Could you check a few things on this model? Use its own coordinates, in mm. A direction names the side the tool comes from. Give positions to 0.01 mm unless a question says otherwise; leave off trailing zeros. Order: outer loops, then holes, each group sorted by start corner. A loop starts at its lowest first (then second) coordinate and runs counter-clockwise, first axis right, second up. Notation, with made-up numbers: (-26.75, 73.25) -> (20.25, 73.25) arc R18 ccw to (20.25, 91.25) -> close; hole circle Ø3 at (2, 4.5). An arc over 180 degrees is marked (long way). Answer as CSV lines item,"result". Start each with the question number.
(1) I want a section at A-A (x = 32). Give the number of separate pieces and of enclosed holes in the cut face, plus the area to 3 significant figures.
(2) On a 3-axis mill with a long thin cutter (end or side, diameter ignored), from which of +Z, -Z, +X, -X, +Y, -Y can I reach the whole of each face in a straight line? I mean faces 1 (the face through (63, 7, 0)), 2 (the face through (2.6, 7, -2)), 3 (the face through (32, 11, 41)), 4 (the face through (45.997, 8.731, 41.789)), 5 (the face through (61.4, 7, 42)). Say none if no direction works.
(3) Will these pins go through, and if not, where does the flat tip stop? pin 1 Ø5 at (x, z) = (38, 33) entering from +Y; pin 2 Ø1.3 at (y, z) = (5, -1) entering from +X; pin 3 Ø5 at (y, z) = (1.5, 18.5) entering from +X; pin 4 Ø1.5 at (y, z) = (1.5, 11) entering from -X.
(4) I want a section at D-D (x = 40). Please give me the cut outline in (y, z), plus the area to 3 significant figures.
(5) I need wall thicknesses on L1, parallel to Z at x = 63, y = 8.1; L2, parallel to Z at x = 44, y = 11.5; L3, parallel to X at y = 12, z = 23.5. Which ranges of each line are inside material? Lowest first, please.
(6) I want a section at B-B (z = 33). Please give me the cut outline in (x, y), plus the area to 3 significant figures.
(7) We'd pull the mould along Z, two halves only. Please class faces 6 (the face through (18.1, 8.19, 41.79)), 7 (the face through (32, 11, -2.6)), 8 (the face through (31.6, 1.6, 10.8)): released by +Z, released by -Z, zero draft, split by the parting line, or undercut.
(8) I want a section at C-C (y = 4.5). Please give me the cut outline in (x, z), plus the area to 3 significant figures.
```python
from build123d import *

# Parameters (mm, degrees)
SKETCH1_W                      = 64
SKETCH1_H                      = 40
BOSS_EXTRUDE1_DEPTH            = 1.6
SKETCH2_R                      = 2.1
CUT_EXTRUDE1_DEPTH             = 76.488807117
LPATTERN1_COUNT                = 2
LPATTERN1_PITCH                = 48
LPATTERN1_COUNT_DIR2           = 5
LPATTERN1_PITCH_DIR2           = 8
EDGE_FLANGE1_STRIP_W           = 8.4
EDGE_FLANGE1_STRIP_H           = 1.6
EDGE_FLANGE1_STRIP_CUT_DEPTH   = 40
EDGE_FLANGE1_STRIP_2_W         = 8.4
EDGE_FLANGE1_STRIP_2_H         = 1.6
EDGE_FLANGE1_STRIP_CUT_2_DEPTH = 40
EDGE_FLANGE1_DEPTH             = 40
EDGE_FLANGE1_BEND_DEPTH        = 40
SKETCH14_R                     = 2.1
CUT_EXTRUDE2_DEPTH             = 77.852130745
LPATTERN2_COUNT                = 5
LPATTERN2_PITCH                = 8
EDGE_FLANGE2_DEPTH             = 58.8
EDGE_FLANGE2_BEND_DEPTH        = 58.8
SKETCH25_R                     = 2.1
CUT_EXTRUDE3_DEPTH             = 80.700690085
LPATTERN3_COUNT                = 7
LPATTERN3_PITCH                = 8
SKETCH26_R                     = 9
SKETCH26_R_2                   = 2
CUT_EXTRUDE4_DEPTH             = 79.255479041


# Sheet-metal steps are written as plain solids
with BuildPart() as part:
    # Sketch1 → Boss-Extrude1 (new body)
    with BuildSketch(Plane(origin=(0, 0, 0), x_dir=(1, 0, 0), z_dir=(0, 1, 0))):
        with Locations((32, -20)):
            Rectangle(SKETCH1_W, SKETCH1_H)
    extrude(amount=BOSS_EXTRUDE1_DEPTH)

    # Sketch2 → Cut-Extrude1 (cut, through all)
    with BuildSketch(Plane(origin=(0, 1.6, 0), x_dir=(1, 0, 0), z_dir=(0, 1, 0))):
        with Locations(Location((8, -4, 0), (0, 0, 270))):
            Circle(SKETCH2_R)
    cut_extrude1 = extrude(amount=-CUT_EXTRUDE1_DEPTH, mode=Mode.SUBTRACT)

    # LPattern1: Cut-Extrude1 2 × 5
    with Locations(*[(i * LPATTERN1_PITCH, 0, j * LPATTERN1_PITCH_DIR2) for i in range(LPATTERN1_COUNT) for j in range(LPATTERN1_COUNT_DIR2) if (i, j) != (0, 0)]):
        add(cut_extrude1, mode=Mode.SUBTRACT)

    # Edge-Flange1 strip (across the edge) → Edge-Flange1 strip cut (cut)
    with BuildSketch(Plane(origin=(64, 1.6, 40), x_dir=(-1, 0, 0), z_dir=(0, 0, -1))):
        with Locations((-1.6, -0.8)):
            Rectangle(EDGE_FLANGE1_STRIP_W, EDGE_FLANGE1_STRIP_H)
    extrude(amount=EDGE_FLANGE1_STRIP_CUT_DEPTH, mode=Mode.SUBTRACT)

    # Edge-Flange1 strip 2 (across the edge) → Edge-Flange1 strip cut 2 (cut)
    with BuildSketch(Plane(origin=(0, 1.6, 0), x_dir=(1, 0, 0), z_dir=(0, 0, 1))):
        with Locations((-1.6, -0.8)):
            Rectangle(EDGE_FLANGE1_STRIP_2_W, EDGE_FLANGE1_STRIP_2_H)
    extrude(amount=EDGE_FLANGE1_STRIP_CUT_2_DEPTH, mode=Mode.SUBTRACT)

    # Edge-Flange1 section (across the edge) → Edge-Flange1 (add)
    with BuildSketch(Plane(origin=(64, 1.6, 40), x_dir=(-1, 0, 0), z_dir=(0, 0, -1))):
        with BuildLine():
            Line((0, 1), (0, 12.9))
            Line((0, 12.9), (1.6, 12.9))
            Line((1.6, 12.9), (1.6, 1))
            ThreePointArc((1.6, 1), (1.892893219, 0.292893219), (2.6, 0))
            Line((2.6, 0), (2.6, -1.6))
            ThreePointArc((2.6, -1.6), (0.761522369, -0.838477631), (0, 1))
        make_face()
    extrude(amount=EDGE_FLANGE1_DEPTH)

    # Edge-Flange1 section 2 (across the edge) → Edge-Flange1 bend (add)
    with BuildSketch(Plane(origin=(0, 1.6, 0), x_dir=(1, 0, 0), z_dir=(0, 0, 1))):
        with BuildLine():
            Line((0, 1), (0, 12.9))
            Line((0, 12.9), (1.6, 12.9))
            Line((1.6, 12.9), (1.6, 1))
            ThreePointArc((1.6, 1), (1.892893219, 0.292893219), (2.6, 0))
            Line((2.6, 0), (2.6, -1.6))
            ThreePointArc((2.6, -1.6), (0.761522369, -0.838477631), (0, 1))
        make_face()
    extrude(amount=EDGE_FLANGE1_BEND_DEPTH)

    # Sketch14 → Cut-Extrude2 (cut, through all)
    with BuildSketch(Plane.ZY):
        with Locations(Location((4, 8.1, 0), (0, 0, 270))):
            Circle(SKETCH14_R)
    cut_extrude2 = extrude(amount=-CUT_EXTRUDE2_DEPTH, mode=Mode.SUBTRACT)

    # LPattern2: Cut-Extrude2 ×5
    with Locations(*[(0, 0, i * LPATTERN2_PITCH) for i in range(1, LPATTERN2_COUNT)]):
        add(cut_extrude2, mode=Mode.SUBTRACT)

    # Edge-Flange2 section (across the edge) → Edge-Flange2 (add)
    with BuildSketch(Plane(origin=(2.6, 1.6, 41), x_dir=(0, 0, -1), z_dir=(1, 0, 0))):
        with BuildLine():
            Line((-1.6, 1), (-1.6, 13))
            Line((-1.6, 13), (0, 13))
            Line((0, 13), (0, 1))
            ThreePointArc((0, 1), (0.292893219, 0.292893219), (1, 0))
            Line((1, 0), (1, -1.6))
            ThreePointArc((1, -1.6), (-0.838477631, -0.838477631), (-1.6, 1))
        make_face()
    extrude(amount=EDGE_FLANGE2_DEPTH)

    # Edge-Flange2 section 2 (across the edge) → Edge-Flange2 bend (add)
    with BuildSketch(Plane(origin=(61.4, 1.6, -1), x_dir=(0, 0, 1), z_dir=(-1, 0, 0))):
        with BuildLine():
            Line((-1.6, 1), (-1.6, 13))
            Line((-1.6, 13), (0, 13))
            Line((0, 13), (0, 1))
            ThreePointArc((0, 1), (0.292893219, 0.292893219), (1, 0))
            Line((1, 0), (1, -1.6))
            ThreePointArc((1, -1.6), (-0.838477631, -0.838477631), (-1.6, 1))
        make_face()
    extrude(amount=EDGE_FLANGE2_BEND_DEPTH)

    # Sketch25 → Cut-Extrude3 (cut, through all)
    with BuildSketch(Plane(origin=(0, 0, -2.6), x_dir=(-1, 0, 0), z_dir=(0, 0, -1))):
        with Locations((-8, 8.1)):
            Circle(SKETCH25_R)
    cut_extrude3 = extrude(amount=-CUT_EXTRUDE3_DEPTH, mode=Mode.SUBTRACT)

    # LPattern3: Cut-Extrude3 ×7
    with Locations(*[(i * LPATTERN3_PITCH, 0, 0) for i in range(1, LPATTERN3_COUNT)]):
        add(cut_extrude3, mode=Mode.SUBTRACT)

    # Sketch26 → Cut-Extrude4 (cut, through all)
    with BuildSketch(Plane.XZ):
        with Locations(Location((32, 20, 0), (0, 0, 270))):
            Circle(SKETCH26_R)
        with Locations(Location((45, 20, 0), (0, 0, 270))):
            Circle(SKETCH26_R_2)
        with Locations(Location((32, 7, 0), (0, 0, 270))):
            Circle(SKETCH26_R_2)
        with Locations(Location((19, 20, 0), (0, 0, 270))):
            Circle(SKETCH26_R_2)
        with Locations(Location((32, 33, 0), (0, 0, 270))):
            Circle(SKETCH26_R_2)
    extrude(amount=-CUT_EXTRUDE4_DEPTH, mode=Mode.SUBTRACT)


solid = part.part
```
Final values:
1,separate pieces,"6"
1,enclosed holes,"0"
1,area,"56.4 mm²"
2,face 1,"-Z, +X, +Y, -Y"
2,face 2,"-Z, -X, +Y, -Y"
2,face 3,"+X, -X, +Y"
2,face 4,"+Z, -Z"
2,face 5,"+Z, +X, +Y, -Y"
3,pin 1,"y = 1.6"
3,pin 2,"x = 61.4"
3,pin 3,"x = 64"
3,pin 4,"x = 0.02"
4,outline,"(0, 0) arc R2.6 ccw to (2.6, -2.6) -> (6, -2.6) -> (6, -1) -> (2.6, -1) arc R1 cw to (1.6, 0) -> (1.6, 15.88) -> (0, 15.88) -> close; (0, 24.12) -> (1.6, 24.12) -> (1.6, 40) arc R1 cw to (2.6, 41) -> (6, 41) -> (6, 42.6) -> (2.6, 42.6) arc R2.6 ccw to (0, 40) -> close; (10.2, -2.6) -> (14.6, -2.6) -> (14.6, -1) -> (10.2, -1) -> close; (10.2, 41) -> (14.6, 41) -> (14.6, 42.6) -> (10.2, 42.6) -> close"
4,area,"84.8 mm²"
5,L1,"0 to 1.9, 6.1 to 9.9, 14.1 to 17.9, 22.1 to 25.9, 30.1 to 33.9, 38.1 to 40"
5,L2,"-2.6 to -1, 41 to 42.6"
5,L3,"0 to 1.6, 62.4 to 64"
6,outline,"(0, 2.6) arc R2.6 ccw to (2.6, 0) -> (30, 0) -> (30, 1.6) -> (2.6, 1.6) arc R1 cw to (1.6, 2.6) -> (1.6, 14.5) -> (0, 14.5) -> close; (34, 0) -> (61.4, 0) arc R2.6 ccw to (64, 2.6) -> (64, 14.5) -> (62.4, 14.5) -> (62.4, 2.6) arc R1 cw to (61.4, 1.6) -> (34, 1.6) -> close"
6,area,"135 mm²"
7,face 6,"zero draft"
7,face 7,"released by -Z"
7,face 8,"undercut"
8,outline,"(0, 0) -> (1.6, 0) -> (1.6, 40) -> (0, 40) -> close; (2.6, -2.6) -> (61.4, -2.6) -> (61.4, -1) -> (2.6, -1) -> close; (2.6, 41) -> (61.4, 41) -> (61.4, 42.6) -> (2.6, 42.6) -> close; (62.4, 0) -> (64, 0) -> (64, 40) -> (62.4, 40) -> close"
8,area,"316 mm²"
